from build123d import *

# Parameters (mm, degrees)
SKETCH7_W               = 22.627416998
SKETCH7_H               = 22.627416998
SKETCH7_R               = 16.1
BOSS_EXTRUDE2_DEPTH     = 8.2
SKETCH1_R               = 2.707265749
SKETCH1_R_2             = 6.25
BOSS_EXTRUDE1_DEPTH     = 5.18
CUT_EXTRUDE1_DEPTH      = 52.274012911
CUT_EXTRUDE1_DEPTH_BACK = 52.274012911
SKETCH6_R               = 1.7
SKETCH9_R               = 2.707265749
SKETCH9_R_2             = 6.25
SKETCH9_R_3             = 1.7
CUT_EXTRUDE2_DEPTH      = 52.274012911
BOSS_EXTRUDE3_START     = 9
SKETCH10_R              = 21
SKETCH10_R_2            = 16.1
BOSS_EXTRUDE3_DEPTH     = 9
CHAMFER1_SIZE           = 1.5
BOSS_EXTRUDE4_START     = 1
SKETCH11_R              = 2.707265749
BOSS_EXTRUDE4_DEPTH     = 1


with BuildPart() as part:
    # Sketch7 → Boss-Extrude2 (new body)
    with BuildSketch(Plane(origin=(0, 0, 0), x_dir=(1, 0, 0), z_dir=(0, 1, 0))):
        Rectangle(SKETCH7_W, SKETCH7_H)
        with Locations(Location((0, 0, 0), (0, 0, 270))):
            Circle(SKETCH7_R)
        Rectangle(SKETCH7_W, SKETCH7_H)
    extrude(amount=BOSS_EXTRUDE2_DEPTH)

    # Sketch1 → Boss-Extrude1 (add)
    with BuildSketch(Plane(origin=(0, 8.2, 0), x_dir=(1, 0, 0), z_dir=(0, 1, 0))):
        with BuildLine():
            Line((15, 25.980762114), (17.5, 30.310889132))
            ThreePointArc((17.5, 30.310889132), (0, 35), (-17.5, 30.310889132))
            Line((-17.5, 30.310889132), (-15, 25.980762114))
            ThreePointArc((-15, 25.980762114), (-25.980762114, 15), (-30, 0))
            Line((-30, 0), (-35, 0))
            ThreePointArc((-35, 0), (-30.310889132, -17.5), (-17.5, -30.310889132))
            Line((-17.5, -30.310889132), (-15, -25.980762114))
            ThreePointArc((-15, -25.980762114), (0, -30), (15, -25.980762114))
            Line((15, -25.980762114), (17.5, -30.310889132))
            ThreePointArc((17.5, -30.310889132), (30.310889132, -17.5), (35, 0))
            Line((35, 0), (30, 0))
            ThreePointArc((30, 0), (25.980762114, 15), (15, 25.980762114))
        make_face()
        with Locations(Location((21.650635095, -12.5, 0), (0, 0, 270))):
            Circle(SKETCH1_R, mode=Mode.SUBTRACT)
        with Locations(Location((-21.650635095, -12.5, 0), (0, 0, 270))):
            Circle(SKETCH1_R, mode=Mode.SUBTRACT)
        with Locations(Location((0, 0, 0), (0, 0, 270))):
            Circle(SKETCH1_R_2, mode=Mode.SUBTRACT)
        with Locations(Location((0, 25, 0), (0, 0, 270))):
            Circle(SKETCH1_R, mode=Mode.SUBTRACT)
    extrude(amount=BOSS_EXTRUDE1_DEPTH)

    # Sketch6 → Cut-Extrude1 (cut, two sides: drawn at the far end of the back side and taken through both)
    with BuildSketch(Plane(origin=(0, 13.38, 0), x_dir=(1, 0, 0), z_dir=(0, 1, 0)).offset(-CUT_EXTRUDE1_DEPTH_BACK)):
        with Locations(Location((0, -9.385, 0), (0, 0, 90))):
            Circle(SKETCH6_R)
        with Locations(Location((-8.127648415, -4.6925, 0), (0, 0, 90))):
            Circle(SKETCH6_R)
        with Locations(Location((-8.127648415, 4.6925, 0), (0, 0, 90))):
            Circle(SKETCH6_R)
        with Locations(Location((0, 9.385, 0), (0, 0, 90))):
            Circle(SKETCH6_R)
        with Locations(Location((8.127648415, 4.6925, 0), (0, 0, 90))):
            Circle(SKETCH6_R)
        with Locations(Location((8.127648415, -4.6925, 0), (0, 0, 90))):
            Circle(SKETCH6_R)
    extrude(amount=CUT_EXTRUDE1_DEPTH + CUT_EXTRUDE1_DEPTH_BACK, mode=Mode.SUBTRACT)

    # Sketch9 → Cut-Extrude2 (cut, through all)
    with BuildSketch(Plane(origin=(0, 13.38, 0), x_dir=(1, 0, 0), z_dir=(0, 1, 0))):
        with Locations(Location((-21.650635095, -12.5, 0), (0, 0, 270))):
            Circle(SKETCH9_R)
        with Locations(Location((0, 0, 0), (0, 0, 270))):
            Circle(SKETCH9_R_2)
        with Locations(Location((21.650635095, -12.5, 0), (0, 0, 270))):
            Circle(SKETCH9_R)
        with Locations(Location((0, 25, 0), (0, 0, 270))):
            Circle(SKETCH9_R)
        with Locations(Location((8.127648415, -4.6925, 0), (0, 0, 90))):
            Circle(SKETCH9_R_3)
        with Locations(Location((8.127648415, 4.6925, 0), (0, 0, 90))):
            Circle(SKETCH9_R_3)
        with Locations(Location((0, 9.385, 0), (0, 0, 90))):
            Circle(SKETCH9_R_3)
        with Locations(Location((-8.127648415, 4.6925, 0), (0, 0, 90))):
            Circle(SKETCH9_R_3)
        with Locations(Location((-8.127648415, -4.6925, 0), (0, 0, 90))):
            Circle(SKETCH9_R_3)
    extrude(amount=-CUT_EXTRUDE2_DEPTH, mode=Mode.SUBTRACT)

    # Sketch10 → Boss-Extrude3 (add)
    with BuildSketch(Plane.XZ.offset(-8.2).offset(BOSS_EXTRUDE3_START)):
        with Locations(Location((0, 0, 0), (0, 0, 90))):
            Circle(SKETCH10_R)
        with Locations(Location((0, 0, 0), (0, 0, 90))):
            Circle(SKETCH10_R_2, mode=Mode.SUBTRACT)
    extrude(amount=-BOSS_EXTRUDE3_DEPTH)

    # Chamfer1
    # the kernel refuses this chamfer: 1.5 mm, written as the material it takes off along each edge
    with BuildSketch(Plane(origin=(0, -0.8, 0), x_dir=(0, 0, 1), z_dir=(1, 0, 0))) as chamfer1_piece_1_section:
        Polygon((16.1, -CHAMFER1_SIZE), (16.1 + CHAMFER1_SIZE, 0), (16.1, 0), align=None)
    chamfer1_piece_1 = revolve(axis=Axis((0, -0.8, 0), (0, -1, 0)), mode=Mode.PRIVATE)
    chamfer1_piece_1 = split(chamfer1_piece_1, bisect_by=Plane(origin=(0, 0, -17.188347783), z_dir=(0, -1, 0)), keep=Keep.TOP, mode=Mode.PRIVATE)
    add(chamfer1_piece_1, mode=Mode.SUBTRACT)

    # Sketch11 → Boss-Extrude4 (add)
    with BuildSketch(Plane.XZ.offset(-8.2).offset(BOSS_EXTRUDE4_START)):
        with BuildLine():
            Line((-35, 0), (-30, 0))
            ThreePointArc((-30, 0), (-25.980762114, -15), (-15, -25.980762114))
            Line((-15, -25.980762114), (-17.5, -30.310889132))
            ThreePointArc((-17.5, -30.310889132), (0, -35), (17.5, -30.310889132))
            Line((17.5, -30.310889132), (15, -25.980762114))
            ThreePointArc((15, -25.980762114), (25.980762114, -15), (30, 0))
            Line((30, 0), (35, 0))
            ThreePointArc((35, 0), (30.310889132, 17.5), (17.5, 30.310889132))
            Line((17.5, 30.310889132), (15, 25.980762114))
            ThreePointArc((15, 25.980762114), (0, 30), (-15, 25.980762114))
            Line((-15, 25.980762114), (-17.5, 30.310889132))
            ThreePointArc((-17.5, 30.310889132), (-30.310889132, 17.5), (-35, 0))
        make_face()
        with Locations(Location((21.650635095, 12.5, 0), (0, 0, 270))):
            Circle(SKETCH11_R, mode=Mode.SUBTRACT)
        with Locations(Location((0, -25, 0), (0, 0, 270))):
            Circle(SKETCH11_R, mode=Mode.SUBTRACT)
        with Locations(Location((-21.650635095, 12.5, 0), (0, 0, 270))):
            Circle(SKETCH11_R, mode=Mode.SUBTRACT)
    extrude(amount=-BOSS_EXTRUDE4_DEPTH)


solid = part.part
Design review of the part built by this model. Coordinates are the model's own, in mm. A direction names the side the tool comes from. Round coordinates to 2 decimals unless told otherwise and drop trailing zeros. Order: outer loops, then holes, each group sorted by start corner. A loop starts at its lowest first (then second) coordinate and runs counter-clockwise, first axis right, second up.
1) Draft analysis for pull direction X (two halves, no side actions). For faces 3 (the cylindrical face through (-30.182, 10.247, 17.722)), 4 (the flat face through (7, 13.38, -3)), 5 (the flat face through (8, 8.2, 5)), 6 (the flat face through (-8, 8.2, 5)), state which applies: released by +X, released by -X, zero draft, split by the parting line, or undercut.
The answers:
face 3: released by -X
face 4: zero draft
face 5: undercut
face 6: undercut
2) Machinability: for faces 1 (the cylindrical face through (6.442, 10.754, -4.471)), 2 (the cylindrical face through (6.442, 3.55, -4.471)), which of the approach directions +Z, -Z, +X, -X, +Y, -Y give a long, thin tool a straight path to every point of the face, cutting with its end or side? Answer none if there is none.
The answers:
face 1: +Y
face 2: -Y
3) For L1, parallel to X at y = 9.35, z = 12.5; L2, parallel to Z at x = -7.5, y = 0.75; L3, parallel to Y at x = 12, z = -22, list the stretches that pass through material, from the lowest coordinate up.
The answers:
L1: x = -32.69 to -24.36, -18.94 to 18.94, 24.36 to 32.69
L2: z = -19.62 to -6.27, -3.11 to 3.11, 6.27 to 19.62
L3: y = 7.2 to 13.38
4) Consider section B-B (y = 3). Count the separate pieces of the cut face and the enclosed holes in it, plus the area to 3 significant figures.
The answers:
separate pieces: 1
enclosed holes: 7
area: 1,210 mm2
5) Clearance check with flat-ended pins moving along their axes: pin 1 Ø5.5 at (x, y) = (-33.5, 9.5) entering from -Z; pin 2 Ø3 at (x, z) = (-8.13, 4.69) entering from -Y; pin 3 Ø8 at (x, y) = (2, 1.5) entering from +Z; pin 4 Ø4.5 at (x, z) = (-21.65, 12.5) entering from -Y. State where each tip first meets the part, or that it passes through.
The answers:
pin 1: stops at z = 0
pin 2: stops at y = 7.2
pin 3: stops at z = 21
pin 4: passes through
6) Consider section D-D (z = 19). State the section outline as (x, y) points, plus the area to 3 significant figures.
The answers:
outline: (-29.39, 7.2) - (-8.94, 7.2) - (-8.94, -0.8) - (8.94, -0.8) - (8.94, 7.2) - (29.39, 7.2) - (29.39, 13.38) - (-29.39, 13.38) - close
area: 506 mm2
